Can you work these out from the model? Positions are in its coordinate system, mm. Coordinates: 2 decimals unless noted, no trailing zeros. Write each loop counter-clockwise with the first axis right and the second up, starting at its lowest first coordinate (ties: lowest second). Pieces come first, ordered by that corner, then holes. Notation, with made-up numbers: (-24, -1.75) - (27, -1.75) arc R20 ccw to (27, 12.25) - close; hole circle Ø3 at (44.5, 58.25). An arc over 180 degrees is marked (long way). One line per question, with ' | ' between items. Start each with the question number.
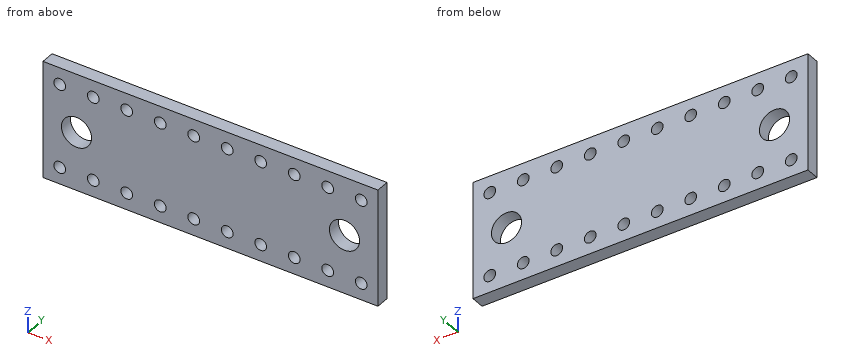
from build123d import *

# Parameters (mm, degrees)
SKETCH1_W               = 100
SKETCH1_H               = 35
BOSS_EXTRUDE1_DEPTH     = 4
CUT_EXTRUDE1_START      = -5
SKETCH2_R               = 1.75
CUT_EXTRUDE1_DEPTH      = 6
LPATTERN1_COUNT         = 10
LPATTERN1_PITCH         = 10
MIRROR1_START           = -5
MIRROR1_COPY_1_SKETCH_R = 1.75
MIRROR1_COPY_1_DEPTH    = 6
MIRROR1_COPY_2_SKETCH_R = 1.75
MIRROR1_COPY_2_DEPTH    = 6
MIRROR1_COPY_3_SKETCH_R = 1.75
MIRROR1_COPY_3_DEPTH    = 6
MIRROR1_COPY_4_SKETCH_R = 1.75
MIRROR1_COPY_4_DEPTH    = 6
MIRROR1_COPY_5_SKETCH_R = 1.75
MIRROR1_COPY_5_DEPTH    = 6
MIRROR1_COPY_6_SKETCH_R = 1.75
MIRROR1_COPY_6_DEPTH    = 6
MIRROR1_COPY_7_SKETCH_R = 1.75
MIRROR1_COPY_7_DEPTH    = 6
MIRROR1_COPY_8_SKETCH_R = 1.75
MIRROR1_COPY_8_DEPTH    = 6
MIRROR1_COPY_9_SKETCH_R = 1.75
MIRROR1_COPY_9_DEPTH    = 6
SKETCH2_3_R             = 4.5
CUT_EXTRUDE3_DEPTH      = 4


with BuildPart() as part:
    # Sketch1 → Boss-Extrude1 (new body)
    with BuildSketch(Plane(origin=(0, 0, 0), x_dir=(1, 0, 0), z_dir=(0, 1, 0))):
        with Locations((50, 17.5)):
            Rectangle(SKETCH1_W, SKETCH1_H)
    extrude(amount=BOSS_EXTRUDE1_DEPTH)

    # Sketch2 → Cut-Extrude1 (cut)
    with BuildSketch(Plane(origin=(0, 4, 0), x_dir=(1, 0, 0), z_dir=(0, 1, 0)).offset(CUT_EXTRUDE1_START)):
        with Locations((5, 30)):
            Circle(SKETCH2_R)
    cut_extrude1 = extrude(amount=CUT_EXTRUDE1_DEPTH, mode=Mode.SUBTRACT)

    # LPattern1: Cut-Extrude1 ×10
    with Locations(*[(i * LPATTERN1_PITCH, 0, 0) for i in range(1, LPATTERN1_COUNT)]):
        add(cut_extrude1, mode=Mode.SUBTRACT)

    # Mirror1: Cut-Extrude1 across plane
    add(cut_extrude1.mirror(Plane(origin=(0, 0, -17.5), x_dir=(1, 0, 0), z_dir=(0, 0, -1))), mode=Mode.SUBTRACT)

    # Mirror1 copy 1 sketch → Mirror1 copy 1 (cut)
    with BuildSketch(Plane(origin=(10, 4, -35), x_dir=(1, 0, 0), z_dir=(0, 1, 0)).offset(MIRROR1_START)):
        with Locations((5, -30)):
            Circle(MIRROR1_COPY_1_SKETCH_R)
    extrude(amount=MIRROR1_COPY_1_DEPTH, mode=Mode.SUBTRACT)

    # Mirror1 copy 2 sketch → Mirror1 copy 2 (cut)
    with BuildSketch(Plane(origin=(20, 4, -35), x_dir=(1, 0, 0), z_dir=(0, 1, 0)).offset(MIRROR1_START)):
        with Locations((5, -30)):
            Circle(MIRROR1_COPY_2_SKETCH_R)
    extrude(amount=MIRROR1_COPY_2_DEPTH, mode=Mode.SUBTRACT)

    # Mirror1 copy 3 sketch → Mirror1 copy 3 (cut)
    with BuildSketch(Plane(origin=(30, 4, -35), x_dir=(1, 0, 0), z_dir=(0, 1, 0)).offset(MIRROR1_START)):
        with Locations((5, -30)):
            Circle(MIRROR1_COPY_3_SKETCH_R)
    extrude(amount=MIRROR1_COPY_3_DEPTH, mode=Mode.SUBTRACT)

    # Mirror1 copy 4 sketch → Mirror1 copy 4 (cut)
    with BuildSketch(Plane(origin=(40, 4, -35), x_dir=(1, 0, 0), z_dir=(0, 1, 0)).offset(MIRROR1_START)):
        with Locations((5, -30)):
            Circle(MIRROR1_COPY_4_SKETCH_R)
    extrude(amount=MIRROR1_COPY_4_DEPTH, mode=Mode.SUBTRACT)

    # Mirror1 copy 5 sketch → Mirror1 copy 5 (cut)
    with BuildSketch(Plane(origin=(50, 4, -35), x_dir=(1, 0, 0), z_dir=(0, 1, 0)).offset(MIRROR1_START)):
        with Locations((5, -30)):
            Circle(MIRROR1_COPY_5_SKETCH_R)
    extrude(amount=MIRROR1_COPY_5_DEPTH, mode=Mode.SUBTRACT)

    # Mirror1 copy 6 sketch → Mirror1 copy 6 (cut)
    with BuildSketch(Plane(origin=(60, 4, -35), x_dir=(1, 0, 0), z_dir=(0, 1, 0)).offset(MIRROR1_START)):
        with Locations((5, -30)):
            Circle(MIRROR1_COPY_6_SKETCH_R)
    extrude(amount=MIRROR1_COPY_6_DEPTH, mode=Mode.SUBTRACT)

    # Mirror1 copy 7 sketch → Mirror1 copy 7 (cut)
    with BuildSketch(Plane(origin=(70, 4, -35), x_dir=(1, 0, 0), z_dir=(0, 1, 0)).offset(MIRROR1_START)):
        with Locations((5, -30)):
            Circle(MIRROR1_COPY_7_SKETCH_R)
    extrude(amount=MIRROR1_COPY_7_DEPTH, mode=Mode.SUBTRACT)

    # Mirror1 copy 8 sketch → Mirror1 copy 8 (cut)
    with BuildSketch(Plane(origin=(80, 4, -35), x_dir=(1, 0, 0), z_dir=(0, 1, 0)).offset(MIRROR1_START)):
        with Locations((5, -30)):
            Circle(MIRROR1_COPY_8_SKETCH_R)
    extrude(amount=MIRROR1_COPY_8_DEPTH, mode=Mode.SUBTRACT)

    # Mirror1 copy 9 sketch → Mirror1 copy 9 (cut)
    with BuildSketch(Plane(origin=(90, 4, -35), x_dir=(1, 0, 0), z_dir=(0, 1, 0)).offset(MIRROR1_START)):
        with Locations((5, -30)):
            Circle(MIRROR1_COPY_9_SKETCH_R)
    extrude(amount=MIRROR1_COPY_9_DEPTH, mode=Mode.SUBTRACT)

    # Sketch2<3> → Cut-Extrude3 (cut)
    with BuildSketch(Plane(origin=(0, 4, 0), x_dir=(1, 0, 0), z_dir=(0, 1, 0))):
        with Locations((10, 17.5)):
            Circle(SKETCH2_3_R)
    cut_extrude3 = extrude(amount=-CUT_EXTRUDE3_DEPTH, mode=Mode.SUBTRACT)

    # Mirror2: Cut-Extrude3 across plane
    add(cut_extrude3.mirror(Plane(origin=(50, 0, 0), x_dir=(0, 0, 1), z_dir=(1, 0, 0))), mode=Mode.SUBTRACT)


solid = part.part
(1) If I drill on probe 1 along Z at (x, y) = (25, 2.8); probe 2 along X at (y, z) = (0.9, -17.5); probe 3 along X at (y, z) = (3.7, -21), over which ranges is the centre line in solid material (lowest first)?
(2) If we section it at C-C on x = 10: List the corners of the cut face in (y, z) for me, plus the area to 3 significant figures.
(3) If we section it at D-D on z = -15: List the corners of the cut face in (x, y) for me, plus the area to 3 significant figures.
(4) If we section it at A-A on x = 65: List the corners of the cut face in (y, z) for me, plus the area to 3 significant figures.
(5) I'm going to push a flat-ended pin straight in: pin 1 (2 mm diameter, centred on x = 75, z = -30, fed in from +Y). Where does the tip first touch, or does it pass through?
(6) If we section it at B-B on y = 1.9: Give the number of separate pieces and of enclosed holes in the cut face, plus the area to 3 significant figures.
Values:
1) probe 1: -35 to -31.75, -28.25 to -6.75, -3.25 to 0 | probe 2: 0 to 5.5, 14.5 to 85.5, 94.5 to 100 | probe 3: 0 to 7.17, 12.83 to 87.17, 92.83 to 100
2) outline: (0, -35) - (4, -35) - (4, -22) - (0, -22) - close; (0, -13) - (4, -13) - (4, 0) - (0, 0) - close | area: 104 mm2
3) outline: (0, 0) - (6.26, 0) - (6.26, 4) - (0, 4) - close; (13.74, 0) - (86.26, 0) - (86.26, 4) - (13.74, 4) - close; (93.74, 0) - (100, 0) - (100, 4) - (93.74, 4) - close | area: 340 mm2
4) outline: (0, -35) - (4, -35) - (4, -31.75) - (0, -31.75) - close; (0, -28.25) - (4, -28.25) - (4, -6.75) - (0, -6.75) - close; (0, -3.25) - (4, -3.25) - (4, 0) - (0, 0) - close | area: 112 mm2
5) pin 1: through
6) separate pieces: 1 | enclosed holes: 22 | area: 3,180 mm2
